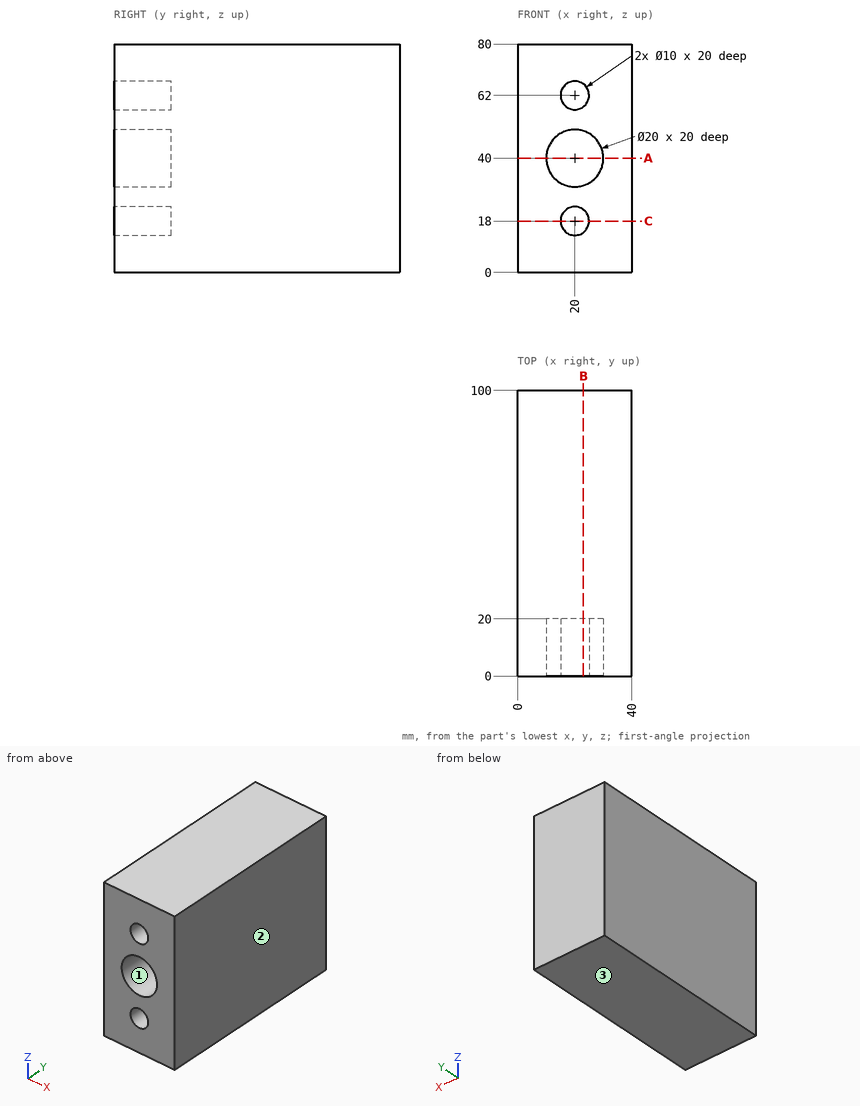
Study the drawing (mm; zero at the part's minimum x, y, z) and answer. Coordinates: 2 decimals unless noted, no trailing zeros. Write each loop counter-clockwise with the first axis right and the second up, starting at its lowest first coordinate (ties: lowest second). Pieces come first, ordered by that corner, then holes. Notation, with made-up numbers: (26.5, -36.5) - (76.5, -36.5) arc R25 cw to (76.5, -18.5) - close; hole circle Ø9 at (-5, -26). An arc over 180 degrees is marked (long way). One line per question, with ' | ' between items.
1) Find section C-C, the plane z = 18. Determine the outline of the cut face in (x, y).
Checks:
outline: (0, 0) - (15, 0) - (15, 20) - (25, 20) - (25, 0) - (40, 0) - (40, 100) - (0, 100) - close
2) Consider probe 1 along X at (y, z) = (12, 40); probe 2 along Z at (x, y) = (17, 12); probe 3 along X at (y, z) = (15, 62). Determine where each line is inside the solid, lowest interval first. Write a range as [from, to].
Checks:
probe 1: [0, 10], [30, 40] | probe 2: [0, 14], [22, 30.46], [49.54, 58], [66, 80] | probe 3: [0, 15], [25, 40]
3) The mould has two halves that part along Z. Classify the marked faces 1, 2 and 3: +Z half, -Z half, draft (parallel to the pull), parting line (faces both ways), or undercut.
Checks:
face 1: undercut | face 2: draft | face 3: -Z half
4) Find section A-A, the plane z = 40. Determine the outline of the cut face in (x, y), and give its area (3 significant figures).
Checks:
outline: (0, 0) - (10, 0) - (10, 20) - (30, 20) - (30, 0) - (40, 0) - (40, 100) - (0, 100) - close | area: 3,600 mm2
5) Find section B-B, the plane x = 23. Determine the outline of the cut face in (y, z).
Checks:
outline: (0, 0) - (100, 0) - (100, 80) - (0, 80) - (0, 66) - (20, 66) - (20, 58) - (0, 58) - (0, 49.54) - (20, 49.54) - (20, 30.46) - (0, 30.46) - (0, 22) - (20, 22) - (20, 14) - (0, 14) - close
6) A flat-ended cylindrical pin translates along its axis: P1, Ø3, axis at x = 21, z = 60.5, coming from the -Y side. Find the tip coordinate at first contact, or state that the pin passes through.
Checks:
P1: y = 20
